Job drawing, mm, ordinate dimensions from the low corner. One solid piece. A direction names the side the tool comes from. Give positions to 0.01 mm unless a question says otherwise; leave off trailing zeros. Order: outer loops, then holes, each group sorted by start corner. A loop starts at its lowest first (then second) coordinate and runs counter-clockwise, first axis right, second up. Notation, with made-up numbers: M 33,38 L 50,38 A28 cw 50,69 Z; hole C -8.75,85.25 d7. An arc over 180 degrees is marked long. Put each result on its own line as item: value. Start each with the question number.
1) Drill centre lines: line 1 (Z direction, x = 39, y = 21); line 2 (X direction, y = 27.5, z = 188); line 3 (Y direction, x = 44, z = 237.5). Where is each one in solid material? Low to high. Write a range as [from, to].
2) Tool access for the marked faces 5 and 6: list every direction of +Z, -Z, +X, -X, +Y, -Y with a clear straight run to the whole face (end or side of a thin tool).
3) Pin check, flat tip, straight feed: pin 1 (4 mm diameter, centred on x = 1.5, z = 206.5, fed in from +Y). Stop position of the tip, or through.
4) Cut at C-C (z = 133.5). Write the cut outline in (x, y).
5) Cut at B-B (y = 14.5). Write the cut outline in (x, z).
6) Two-plate mould, pull along Z, no slides. Class the marked faces 1, 2, 3 and 4: released by +Z, released by -Z, zero draft, split by the parting line, or undercut.
7) Cut at A-A (x = 33.5). Write the cut outline in (y, z), and give its area (3 significant figures).
8) Cut at D-D (x = 13.5). Write the cut outline in (y, z).
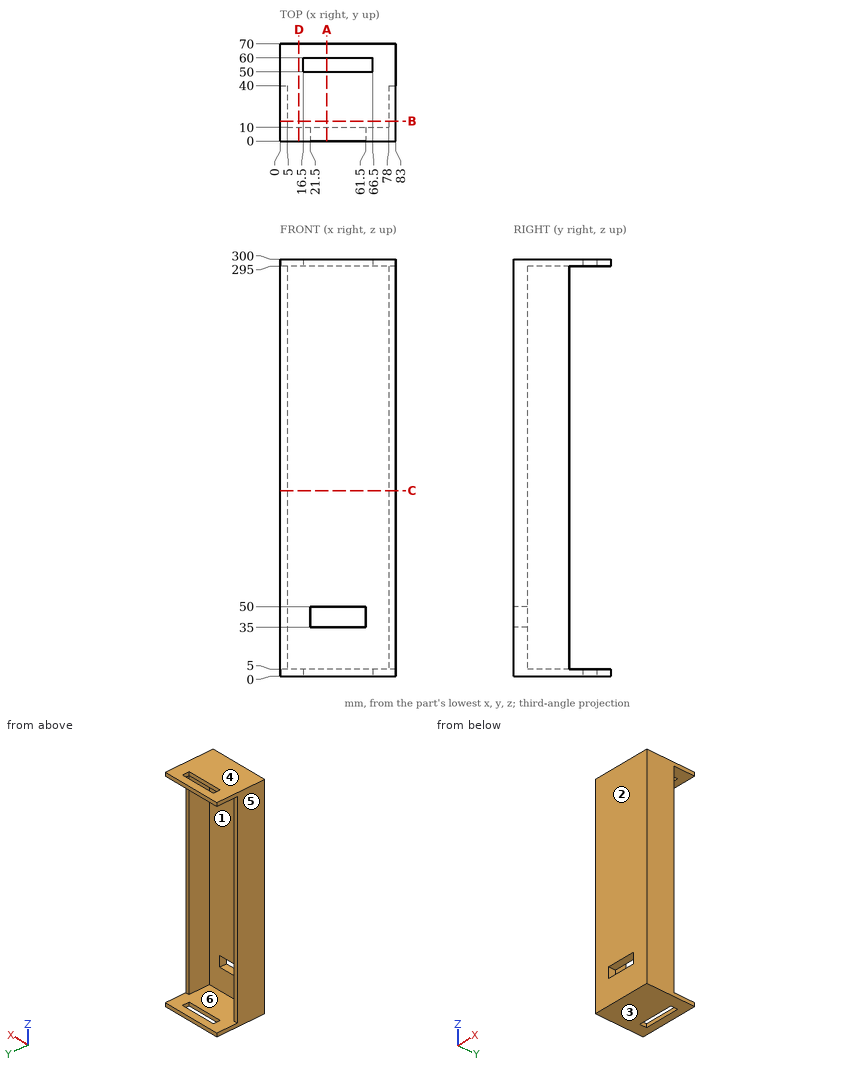
Solution:
1. line 1: [0, 5], [295, 300]
1. line 2: [0, 5], [78, 83]
1. line 3: [0, 10]
2. face 5: +Z, -Z, -X, +Y, -Y
2. face 6: +Y
3. pin 1: y = 40
4. outline: M 0,0 L 83,0 L 83,40 L 78,40 L 78,10 L 5,10 L 5,40 L 0,40 Z
5. outline: M 0,0 L 83,0 L 83,300 L 0,300 Z; hole M 5,5 L 78,5 L 78,295 L 5,295 Z
6. face 1: undercut
6. face 2: zero draft
6. face 3: released by -Z
6. face 4: released by +Z
7. outline: M 0,0 L 50,0 L 50,5 L 10,5 L 10,35 L 0,35 Z; M 0,50 L 10,50 L 10,295 L 50,295 L 50,300 L 0,300 Z; M 60,0 L 70,0 L 70,5 L 60,5 Z; M 60,295 L 70,295 L 70,300 L 60,300 Z
7. area: 3,350 mm²
8. outline: M 0,0 L 70,0 L 70,5 L 10,5 L 10,295 L 70,295 L 70,300 L 0,300 Z
